Geometry check sheet. Reference: the model listing, model coordinates, mm. Face numbers are marked on the shaded views. A direction names the side the tool comes from. Give positions to 0.01 mm unless a question says otherwise; leave off trailing zeros. Write each loop counter-clockwise with the first axis right and the second up, starting at its lowest first coordinate (ties: lowest second). Pieces come first, ordered by that corner, then holes. Notation, with made-up numbers: (-15, 80.25) - (-5, 80.25) arc R19 ccw to (-5, 111.25) - close; hole circle Ø3 at (38.25, 26.25). An arc over 180 degrees is marked (long way). Write item = value, one per line. Start each with the question number.
(1) Section check B-B, the plane x = -1. Enter the section's corners in (y, z), plus the area to 3 significant figures.
(2) Access from +Z, -Z, +X, -X, +Y, -Y to the whole of each face (thin tool, end or side, straight path). Record for the marked faces 1 and 2.
(3) Thickness scan on L1, parallel to Y at x = 3, z = -20.5; L2, parallel to Y at x = 2, z = 30.5. Record the ranges inside material, lowest first.
(4) Section check C-C, the plane z = -17. Enter the section's corners in (x, y).
(5) Section check D-D, the plane x = 16. Enter the section's corners in (y, z).
(6) Section check A-A, the plane x = -6.5. Enter the section's corners in (y, z).
(7) Draft check along Z on the marked faces 3, 4 and 5. Enter one of: pulls with the +Z half, pulls with the -Z half, needs draft (parallel to the pull), parting line crosses it, or undercut.
(8) Depth check by flat-ended pin: pin 1 Ø1.5 at (x, y) = (-2.5, -2.5) entering from +Z; pin 2 Ø3 at (x, y) = (-13.5, -12.5) entering from +Z; pin 3 Ø19 at (x, z) = (6.5, 7.5) entering from -Y; pin 4 Ø5 at (x, z) = (-11, -31.5) entering from -Y. Enter the tip coordinate at first touch or a pass-through.
```python
from build123d import *

# Parameters (mm, degrees)
SKETCH1_W                        = 38.1
SKETCH1_H                        = 44.45
BASE_FLANGE1_DEPTH               = 4.2672
EDGE_FLANGE1_STRIP_CUT_DEPTH     = 38.1
EDGE_FLANGE1_DEPTH               = 38.1
EDGE_FLANGE2_STRIP_CUT_DEPTH     = 38.1
EDGE_FLANGE2_DEPTH               = 38.1
CHAMFER1_SIZE                    = 6.35
F_17_64_0_26563_DIAMETER_HOLE1_D = 6.747002


# Sheet-metal steps are written as plain solids
with BuildPart() as part:
    # Sketch1 → Base-Flange1 (new body)
    with BuildSketch(Plane(origin=(0, 0, 0), x_dir=(1, 0, 0), z_dir=(0, 1, 0))):
        Rectangle(SKETCH1_W, SKETCH1_H)
    extrude(amount=-BASE_FLANGE1_DEPTH)

    # Edge-Flange1 strip (across the edge) → Edge-Flange1 strip cut (cut)
    with BuildSketch(Plane(origin=(19.05, -4.2672, 22.225), x_dir=(0, -0.96592582628907, -0.2588190451025146), z_dir=(-1, 0, 0))):
        Polygon((-9.522131081, 19.049882248), (-4.052559965, -1.362835054), (0.069238721, -0.258402425), (-5.400332395, 20.154314877), align=None)
    extrude(amount=EDGE_FLANGE1_STRIP_CUT_DEPTH, mode=Mode.SUBTRACT)

    # Edge-Flange1 section (across the edge) → Edge-Flange1 (add)
    with BuildSketch(Plane(origin=(19.05, -4.2672, 22.225), x_dir=(0, -0.96592582628907, -0.2588190451025146), z_dir=(-1, 0, 0))):
        with BuildLine():
            Line((-4.2672, 0.267517875), (-4.2672, 50.17300498))
            Line((-4.2672, 50.17300498), (0, 50.17300498))
            Line((0, 50.17300498), (0, 0.267517875))
            ThreePointArc((0, 0.267517875), (0.017384042, 0.002288653), (0.069238721, -0.258402425))
            Line((0.069238721, -0.258402425), (-4.052559965, -1.362835054))
            ThreePointArc((-4.052559965, -1.362835054), (-4.213309471, -0.554692715), (-4.2672, 0.267517875))
        make_face()
    extrude(amount=EDGE_FLANGE1_DEPTH)

    # Edge-Flange2 strip (across the edge) → Edge-Flange2 strip cut (cut)
    with BuildSketch(Plane(origin=(-19.05, -4.2672, -22.225), x_dir=(0, -0.9961946980917461, 0.08715574274765156), z_dir=(1, 0, 0))):
        Polygon((-6.085074523, 20.592090897), (-4.243229642, -0.460292419), (0.007732373, -0.088381433), (-1.834112507, 20.964001883), align=None)
    extrude(amount=EDGE_FLANGE2_STRIP_CUT_DEPTH, mode=Mode.SUBTRACT)

    # Edge-Flange2 section (across the edge) → Edge-Flange2 (add)
    with BuildSketch(Plane(origin=(-19.05, -4.2672, -22.225), x_dir=(0, -0.9961946980917461, 0.08715574274765156), z_dir=(1, 0, 0))):
        with BuildLine():
            Line((-4.2672, 0.088719036), (-4.2672, 50.38333524))
            Line((-4.2672, 50.38333524), (0, 50.38333524))
            Line((0, 50.38333524), (0, 0.088719036))
            ThreePointArc((0, 0.088719036), (0.001934014, 8.4441e-05), (0.007732373, -0.088381433))
            Line((0.007732373, -0.088381433), (-4.243229642, -0.460292419))
            ThreePointArc((-4.243229642, -0.460292419), (-4.261204557, -0.186048209), (-4.2672, 0.088719036))
        make_face()
    extrude(amount=EDGE_FLANGE2_DEPTH)

    # Chamfer1
    chamfer1_edges = [part.edges().sort_by_distance(p)[0] for p in [
        (19.05, -15.192029896, 71.240617608),
        (-19.05, -15.192029896, 71.240617608),
        (-19.05, -6.532915997, -72.602566931),
        (19.05, -6.532915997, -72.602566931),
    ]]
    chamfer(chamfer1_edges, length=CHAMFER1_SIZE)

    # 17/64 (0.26563) Diameter Hole1 (through all)
    with Locations(Plane(origin=(0, 5.696696884, 1.52642533), x_dir=(1, 0, 0), z_dir=(0, 0.9659258262890699, 0.25881904510251463))):
        with Locations((0, -35.539651994), (0, -60.939651994)):
            Hole(F_17_64_0_26563_DIAMETER_HOLE1_D / 2)


solid = part.part
```
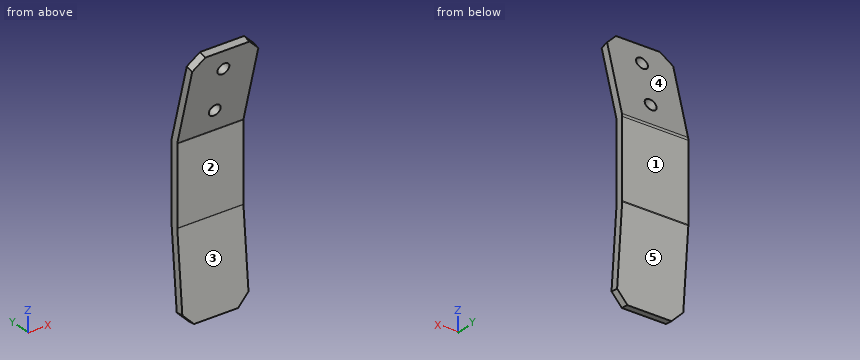
Model answer:
q1.outline = (-17.25, 70.69) - (-15.03, 62.4) - (-10.91, 63.5) - (-13.13, 71.79) - close; (-13.36, 56.17) - (-8.46, 37.86) - (-4.34, 38.97) - (-9.24, 57.28) - close; (-8.66, -72.42) - (-4.41, -72.79) - (-0.02, -22.69) arc R6.3 ccw to (0, -22.14) - (0, 21.96) arc R6.3 ccw to (-0.21, 23.59) - (-2.67, 32.74) - (-6.79, 31.64) - (-4.34, 22.48) arc R2.03 cw to (-4.27, 21.96) - (-4.27, -22.14) arc R2.03 cw to (-4.27, -22.31) - close
q1.area = 567 mm²
q2.face_1 = +Z, -Z, +X, -X, +Y
q2.face_2 = +X, -X, -Y
q3.L1 = -4.27 to 0
q3.L2 = -6.48 to -2.07
q4.outline = (-19.05, -4.27) - (19.05, -4.27) - (19.05, 0) - (-19.05, 0) - close
q5.outline = (-16.4, 67.5) - (-4.34, 22.48) arc R2.03 cw to (-4.27, 21.96) - (-4.27, -22.14) arc R2.03 cw to (-4.27, -22.31) - (-8.37, -69.13) - (-4.12, -69.5) - (-0.02, -22.69) arc R6.3 ccw to (0, -22.14) - (0, 21.96) arc R6.3 ccw to (-0.21, 23.59) - (-12.28, 68.61) - close
q6.outline = (-17.25, 70.69) - (-4.34, 22.48) arc R2.03 cw to (-4.27, 21.96) - (-4.27, -22.14) arc R2.03 cw to (-4.27, -22.31) - (-8.66, -72.42) - (-4.41, -72.79) - (-0.02, -22.69) arc R6.3 ccw to (0, -22.14) - (0, 21.96) arc R6.3 ccw to (-0.21, 23.59) - (-13.13, 71.79) - close
q7.face_3 = undercut
q7.face_4 = pulls with the +Z half
q7.face_5 = pulls with the -Z half
q8.pin_1 = 34.31
q8.pin_2 = 71.79
q8.pin_3 = -4.27
q8.pin_4 = -5.3
